from build123d import *

# Parameters (mm, degrees)
F0_R     = 177.8
F0_R_2   = 22.86
F1_DEPTH = 152.4
F2_R     = 152.4
F2_R_2   = 76.2
F3_DEPTH = 101.6
F4_R     = 177.8
F4_R_2   = 152.4
F5_DEPTH = 50.8


with BuildPart() as f1:
    # F0 (on Top) → F1 (new body)
    with BuildSketch(Plane.XY):
        Circle(F0_R)
        with Locations((-98.986704, -57.15)):
            Circle(F0_R_2, mode=Mode.SUBTRACT)
        with Locations((98.986704, -57.15)):
            Circle(F0_R_2, mode=Mode.SUBTRACT)
        with BuildLine():
            ThreePointArc((12.7, 35.921024), (31.10852, 21.997045), (38.1, 0))
            ThreePointArc((38.1, 0), (-21.997045, -31.10852), (-12.7, 35.921024))
            Line((-12.7, 35.921024), (-12.7, 50.8))
            Line((-12.7, 50.8), (12.7, 50.8))
            Line((12.7, 50.8), (12.7, 35.921024))
        make_face(mode=Mode.SUBTRACT)
        with Locations((0, 114.3)):
            Circle(F0_R_2, mode=Mode.SUBTRACT)
    extrude(amount=F1_DEPTH)

    # F2 (on face) → F3 (cut)
    with BuildSketch(Plane.XY.offset(152.4)):
        Circle(F2_R)
        Circle(F2_R_2, mode=Mode.SUBTRACT)
    extrude(amount=-F3_DEPTH, mode=Mode.SUBTRACT)

    # F4 (on face) → F5 (cut)
    with BuildSketch(Plane.XY.offset(152.4)):
        Circle(F4_R)
        Circle(F4_R_2, mode=Mode.SUBTRACT)
    extrude(amount=-F5_DEPTH, mode=Mode.SUBTRACT)


solid = f1.part
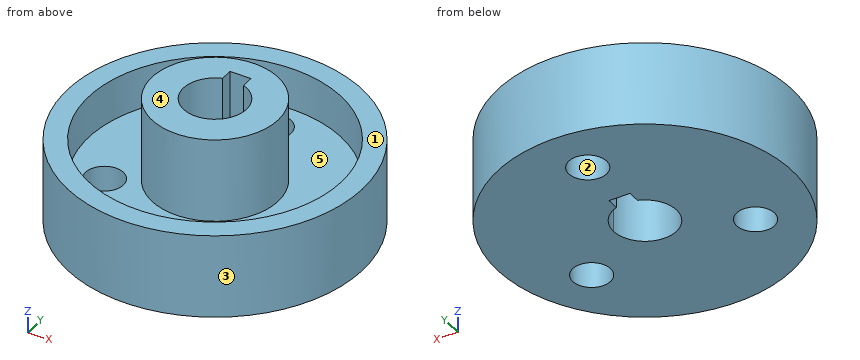
Design review of the part built by this model. Coordinates are the model's own, in mm. Face numbers are marked on the shaded views. A direction names the side the tool comes from. Coordinates: 2 decimals unless noted, no trailing zeros. Write each loop counter-clockwise with the first axis right and the second up, starting at its lowest first coordinate (ties: lowest second). Pieces come first, ordered by that corner, then holes. Notation, with made-up numbers: (28.5, -16) - (80.5, -16) arc R25 ccw to (80.5, 5) - close; hole circle Ø1 at (-11, 11). An arc over 180 degrees is marked (long way). Use one line per item in the form item = value.
Q1. The part is to be moulded in two halves that separate along X. For the marked faces 3, 4 and 5, say which applies: +X half, -X half, draft (parallel to the pull), parting line (faces both ways), or undercut.
Taken from the geometry:
face_3 = parting line
face_4 = draft
face_5 = undercut
Q2. Consider section D-D (x = 114.5). Write out the cut boundary in (y, z).
Taken from the geometry:
outline = (-136.02, 0) - (-73.94, 0) - (-73.94, 50.8) - (-100.58, 50.8) - (-100.58, 101.6) - (-136.02, 101.6) - close; (-40.36, 0) - (136.02, 0) - (136.02, 101.6) - (100.58, 101.6) - (100.58, 50.8) - (-40.36, 50.8) - close
Q3. Consider section B-B (x = 0). Write out the cut boundary in (y, z), plus the area to 3 significant figures.
Taken from the geometry:
outline = (-177.8, 0) - (-38.1, 0) - (-38.1, 152.4) - (-76.2, 152.4) - (-76.2, 50.8) - (-152.4, 50.8) - (-152.4, 101.6) - (-177.8, 101.6) - close; (50.8, 0) - (91.44, 0) - (91.44, 50.8) - (76.2, 50.8) - (76.2, 152.4) - (50.8, 152.4) - close; (137.16, 0) - (177.8, 0) - (177.8, 101.6) - (152.4, 101.6) - (152.4, 50.8) - (137.16, 50.8) - close
area = 20,300 mm^2
Q4. Consider section A-A (z = 62.5). Write out the cut boundary in (x, y).
Taken from the geometry:
outline = circle Ø355.6 at (0, 0); circle Ø152.4 at (0, 0); hole circle Ø304.8 at (0, 0); hole (-12.7, 35.92) arc R38.1 ccw (long way) to (38.1, 0) arc R38.1 ccw to (12.7, 35.92) - (12.7, 50.8) - (-12.7, 50.8) - close
Q5. For probe 1 along Y at (x, z) = (0, 35); probe 2 along X at (y, z) = (50, 96.5); probe 3 along X at (y, z) = (-57, 13), list the stretches that pass through material, from the lowest coordinate up.
Taken from the geometry:
probe_1 = -177.8 to -38.1, 50.8 to 91.44, 137.16 to 177.8
probe_2 = -170.62 to -143.96, -57.5 to -12.7, 12.7 to 57.5, 143.96 to 170.62
probe_3 = -168.42 to -121.85, -76.13 to 76.13, 121.85 to 168.42
Q6. Machinability: for the marked faces 1 and 2, which of the approach directions +Z, -Z, +X, -X, +Y, -Y give a long, thin tool a straight path to every point of the face, cutting with its end or side? Answer none if there is none.
Taken from the geometry:
face_1 = +Z
face_2 = +Z, -Z
Q7. Insertion check: pin 1 Ø3 at (x, y) = (38, 108) entering from -Z; pin 2 Ø10 at (x, z) = (-42, 16.5) entering from +Y; pin 3 Ø4.5 at (y, z) = (42, 107) entering from +X; pin 4 Ø1 at (x, z) = (-105, 56) entering from +Y. Each pin has a flat end and moves straight along its axis. Give the tip position at first contact, or say it passes through.
Taken from the geometry:
pin_1 = 0
pin_2 = 173.91
pin_3 = 65.01
pin_4 = 143.85
Q8. Consider section C-C (y = 8). Write out the cut boundary in (x, z).
Taken from the geometry:
outline = (-177.62, 0) - (-37.25, 0) - (-37.25, 152.4) - (-75.78, 152.4) - (-75.78, 50.8) - (-152.19, 50.8) - (-152.19, 101.6) - (-177.62, 101.6) - close; (37.25, 0) - (177.62, 0) - (177.62, 101.6) - (152.19, 101.6) - (152.19, 50.8) - (75.78, 50.8) - (75.78, 152.4) - (37.25, 152.4) - close
